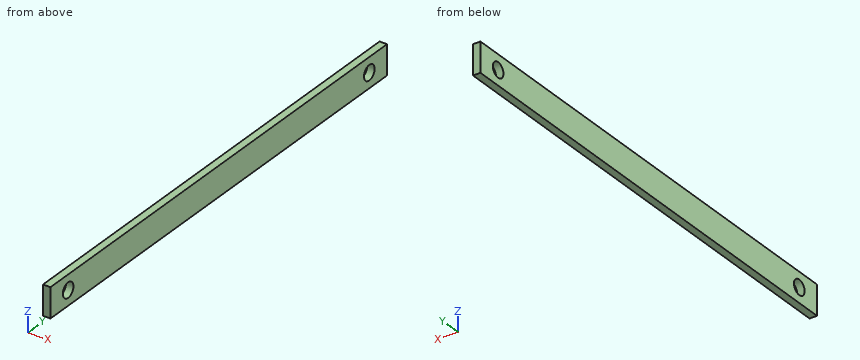
```python
from build123d import *

# Parameters (mm, degrees)
SKETCH1_W           = 12
SKETCH1_H           = 190
BOSS_EXTRUDE1_DEPTH = 3
SKETCH2_R           = 3
CUT_EXTRUDE1_DEPTH  = 3


with BuildPart() as part:
    # Sketch1 → Boss-Extrude1 (new body)
    with BuildSketch(Plane(origin=(0, 0, 0), x_dir=(0, 0, -1), z_dir=(1, 0, 0))):
        Rectangle(SKETCH1_W, SKETCH1_H)
    extrude(amount=BOSS_EXTRUDE1_DEPTH)

    # Sketch2 → Cut-Extrude1 (cut)
    with BuildSketch(Plane.ZY):
        with Locations((0, 85)):
            Circle(SKETCH2_R)
        with Locations((0, -85)):
            Circle(SKETCH2_R)
    extrude(amount=-CUT_EXTRUDE1_DEPTH, mode=Mode.SUBTRACT)


solid = part.part
```
Part model, mm, in its own coordinate system. Coordinates: 2 decimals unless noted, no trailing zeros. Loops run counter-clockwise (first coordinate to the right, second up) from the corner with the lowest first, then second, coordinate; pieces in that order, holes last. Notation, with made-up numbers: (22.25, -22) - (55.25, -22) arc R28 ccw to (55.25, 15) - close; hole circle Ø5 at (47.5, 22.5). An arc over 180 degrees is marked (long way). Write item = value, one per line. Start each with the question number.
Item 1: Cut at B-B, the plane z = 0. Give the cut face in (x, y), and give its area (3 significant figures).
Item 2: Cut at A-A, the plane y = -85. Give the cut face in (x, z).
Item 3: Cut at C-C, the plane x = 2.2. Give the cut face in (y, z).
Item 4: Wall check: L1, parallel to Y at x = 2.2, z = 0; L2, parallel to Y at x = 2.1, z = 1.25; L3, parallel to Z at x = 1.9, y = 85.5. Give the ranges that are in metal, low to high. Write a range as from..to.
The answers:
q1.outline = (0, -95) - (3, -95) - (3, -88) - (0, -88) - close; (0, -82) - (3, -82) - (3, 82) - (0, 82) - close; (0, 88) - (3, 88) - (3, 95) - (0, 95) - close
q1.area = 534 mm2
q2.outline = (0, -6) - (3, -6) - (3, -3) - (0, -3) - close; (0, 3) - (3, 3) - (3, 6) - (0, 6) - close
q3.outline = (-95, -6) - (95, -6) - (95, 6) - (-95, 6) - close; hole circle Ø6 at (-85, 0); hole circle Ø6 at (85, 0)
q4.L1 = -95..-88, -82..82, 88..95
q4.L2 = -95..-87.73, -82.27..82.27, 87.73..95
q4.L3 = -6..-2.96, 2.96..6
